The figure shows three views and two pictorial views of one solid part (mm, origin at its lowest corner). Answer the questions. A direction names the side the tool comes from. Coordinates: 2 decimals unless noted, no trailing zeros. Loops run counter-clockwise (first coordinate to the right, second up) from the corner with the lowest first, then second, coordinate; pieces in that order, holes last. Notation, with made-up numbers: M 20.5,57 L 43.5,57 A13 cw 43.5,81 Z; hole C 82.5,-5 d5. An arc over 180 degrees is marked long. Return JSON: item names as keys, results as strings. Group by question number.
1. Given P1, Ø8, axis at x = 55, y = 57.5, coming from the +Z side; P2, Ø11, axis at y = 16, z = 4, coming from the -X side; P3, Ø5, axis at x = 22.5, z = 36, coming from the +Y side, each flat-ended and moving along its own axis, determine where each tip first touches the part or whether it passes through.
2. Straight lines are drawn through the part: L1, parallel to X at y = 69, z = 81.5; L2, parallel to X at y = 60.5, z = 4; L3, parallel to Y at x = 11, z = 39.5. For each, find the intervals that lie inside material, in ascending order. Write a range as from..to.
3. Section A-A (y = 60) is taken. Write down the section's boundary in (x, z), then the cut area to 3 significant figures.
4. Section B-B (x = 67) is taken. Write down the section's boundary in (y, z), then the cut area to 3 significant figures.
5. Section C-C (z = 67.5) is taken. Write down the section's boundary in (x, y), then the cut area to 3 significant figures.
6. Section D-D (z = 46.5) is taken. Write down the section's boundary in (x, y).
7. Which of the six approach directions +Z, -Z, +X, -X, +Y, -Y give full straight-line access (tool end or side, diameter ignored) to the marked faces 1 and 2?
8. The mould has two halves that part along X. Classify the marked faces 3, 4 and 5: pulls with the +X half, pulls with the -X half, needs draft (parallel to the pull), parting line crosses it, or undercut.
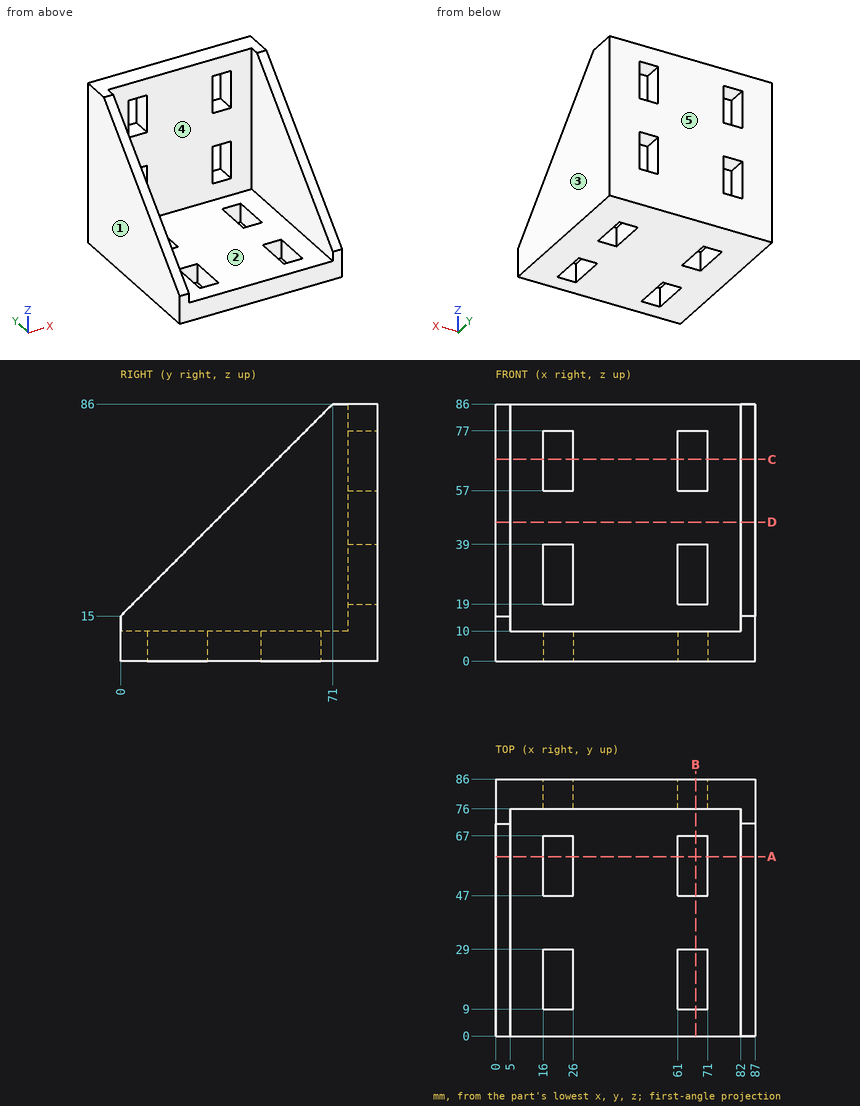
Worked out:
{
 "1": {"P1": "z = 10", "P2": "x = 0", "P3": "through"},
 "2": {"L1": "0..5, 82..87", "L2": "0..16, 26..61, 71..87", "L3": "76..86"},
 "3": {"outline": "M 0,0 L 16,0 L 16,10 L 5,10 L 5,75 L 0,75 Z; M 26,0 L 61,0 L 61,10 L 26,10 Z; M 71,0 L 87,0 L 87,75 L 82,75 L 82,10 L 71,10 Z", "area": "1,320 mm^2"},
 "4": {"outline": "M 0,0 L 9,0 L 9,10 L 0,10 Z; M 29,0 L 47,0 L 47,10 L 29,10 Z; M 67,0 L 86,0 L 86,19 L 76,19 L 76,10 L 67,10 Z; M 76,39 L 86,39 L 86,57 L 76,57 Z; M 76,77 L 86,77 L 86,86 L 76,86 Z", "area": "820 mm^2"},
 "5": {"outline": "M 0,52.5 L 5,52.5 L 5,76 L 16,76 L 16,86 L 0,86 Z; M 26,76 L 61,76 L 61,86 L 26,86 Z; M 71,76 L 82,76 L 82,52.5 L 87,52.5 L 87,86 L 71,86 Z", "area": "905 mm^2"},
 "6": {"outline": "M 0,31.5 L 5,31.5 L 5,76 L 82,76 L 82,31.5 L 87,31.5 L 87,86 L 0,86 Z"},
 "7": {"face 1": "+Z, -Z, -X, +Y, -Y", "face 2": "+Z, -Y"},
 "8": {"face 3": "pulls with the +X half", "face 4": "undercut", "face 5": "needs draft"}
}
